Can you work these out from the drawing? Everything is in mm from the part's minimum corner. A direction names the side the tool comes from. Round coordinates to 2 decimals unless told otherwise and drop trailing zeros. Order: outer loops, then holes, each group sorted by start corner. A loop starts at its lowest first (then second) coordinate and runs counter-clockwise, first axis right, second up. Notation, with made-up numbers: (80, 70.25) -> (130, 70.25) arc R21 cw to (130, 98.25) -> close; hole circle Ø6 at (-32.5, 86.25). An arc over 180 degrees is marked (long way). One line per item, written item: value.
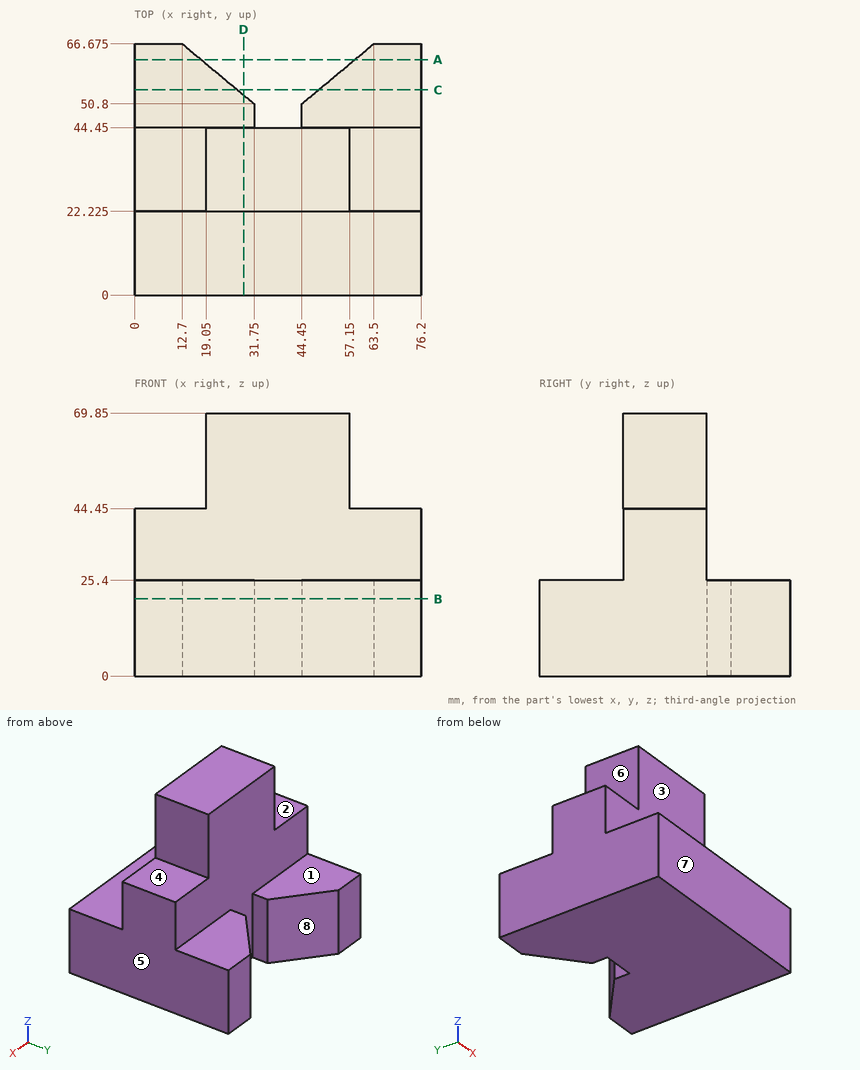
Q1. Which directions (+Z, -Z, +X, -X, +Y, -Y) give clear straight access to the entire face, cutting with the end or side of a thin tool? Please do the marked faces 1, 2, 3 and 4.
Answers:
face 1: +Z, +X, -X, +Y
face 2: +Z, -X, +Y, -Y
face 3: +Z, +X, -X, -Y
face 4: +Z, +X, +Y, -Y
Q2. For P1, Ø6.5, axis at x = 19, y = 53.5, coming from the +Z side; P2, Ø21, axis at x = 7, y = 31, coming from the +Z side; P3, Ø6.5, axis at y = 33.5, z = 57, coming from the -X side, each with a flat end and sliding along its axis, tell me the tip position at first contact or that it passes through.
Answers:
P1: z = 25.4
P2: z = 44.45
P3: x = 19.05
Q3. I want a section at A-A on y = 62.5. Write out the boundary of the cut face in (x, z).
Answers:
outline: (0, 0) -> (17.71, 0) -> (17.71, 25.4) -> (0, 25.4) -> close; (58.49, 0) -> (76.2, 0) -> (76.2, 25.4) -> (58.49, 25.4) -> close
Q4. I want a section at B-B on z = 20.5. Write out the boundary of the cut face in (x, y) (3 decimals).
Answers:
outline: (0, 0) -> (76.2, 0) -> (76.2, 66.675) -> (63.5, 66.675) -> (44.45, 50.8) -> (44.45, 44.45) -> (31.75, 44.45) -> (31.75, 50.8) -> (12.7, 66.675) -> (0, 66.675) -> close
Q5. If we mould it in two halves opening along X, with no side actions, what happens to the marked faces 5, 6, 7 and 8? For each: pulls with the +X half, pulls with the -X half, needs draft (parallel to the pull), parting line crosses it, or undercut.
Answers:
face 5: pulls with the +X half
face 6: pulls with the -X half
face 7: needs draft
face 8: undercut
Q6. I want a section at C-C on y = 54.5. Write out the boundary of the cut face in (x, z).
Answers:
outline: (0, 0) -> (27.31, 0) -> (27.31, 25.4) -> (0, 25.4) -> close; (48.89, 0) -> (76.2, 0) -> (76.2, 25.4) -> (48.89, 25.4) -> close
Q7. I need wall thicknesses on line 1 along X through (y, z) = (50, 7); line 2 along Z through (x, y) = (50, 48); line 3 along Z through (x, y) = (69.5, 25.5). Which ranges of each line are inside material? Lowest first, please.
Answers:
line 1: 0 to 31.75, 44.45 to 76.2
line 2: 0 to 25.4
line 3: 0 to 44.45
Q8. I want a section at D-D on x = 29. Write out the boundary of the cut face in (y, z) (3 decimals), then the cut area to 3 significant figures.
Answers:
outline: (0, 0) -> (53.092, 0) -> (53.092, 25.4) -> (44.45, 25.4) -> (44.45, 69.85) -> (22.225, 69.85) -> (22.225, 25.4) -> (0, 25.4) -> close
area: 2,340 mm2
